from build123d import *

# Parameters (mm, degrees)
SKIZZE1_W                       = 155
SKIZZE1_H                       = 18
AUFSATZ_LINEAR_AUSTRAGEN1_DEPTH = 4
SCHNITT_LINEAR_AUSTRAGEN1_DEPTH = 4
LINEARES_MUSTER1_COUNT          = 22
LINEARES_MUSTER1_PITCH          = 6.379656485
SCHNITT_LINEAR_AUSTRAGEN2_REACH = 6
SKIZZE3_W                       = 115
SKIZZE3_H                       = 4.1
SCHNITT_LINEAR_AUSTRAGEN3_REACH = 6
SKIZZE4_W                       = 3.6
SKIZZE4_H                       = 5


with BuildPart() as part:
    # Skizze1 → Aufsatz-Linear austragen1 (new body)
    with BuildSketch(Plane.XY):
        with Locations((77.5, 9)):
            Rectangle(SKIZZE1_W, SKIZZE1_H)
    extrude(amount=AUFSATZ_LINEAR_AUSTRAGEN1_DEPTH)

    # Skizze2 → Schnitt-Linear austragen1 (cut)
    with BuildSketch(Plane.XY.offset(4)):
        Polygon((0, 13), (1, 13), (2.819851171, 18), (0, 18), align=None)
        Polygon((3.819851171, 18), (5.639702343, 13), (6.639702343, 13), (6.639702343, 18), align=None)
    schnitt_linear_austragen1 = extrude(amount=-SCHNITT_LINEAR_AUSTRAGEN1_DEPTH, mode=Mode.SUBTRACT)

    # Lineares Muster1: Schnitt-Linear austragen1 ×22
    with Locations(*[(i * LINEARES_MUSTER1_PITCH, 0, 0) for i in range(1, LINEARES_MUSTER1_COUNT)]):
        add(schnitt_linear_austragen1, mode=Mode.SUBTRACT)

    # Skizze3 → Schnitt-Linear austragen2 (cut, up to next)
    with BuildSketch(Plane.XY.offset(4), mode=Mode.PRIVATE) as schnitt_linear_austragen2_sk1:
        with Locations((64.227564671, 6.05)):
            Rectangle(SKIZZE3_W, SKIZZE3_H)
    schnitt_linear_austragen2_tool1 = extrude(schnitt_linear_austragen2_sk1.sketch, amount=-SCHNITT_LINEAR_AUSTRAGEN2_REACH, mode=Mode.PRIVATE) & part.part
    add(schnitt_linear_austragen2_tool1.solids().sort_by_distance((64.227565, 6.05, 4))[0], mode=Mode.SUBTRACT)

    # Skizze4 → Schnitt-Linear austragen3 (cut, up to next)
    with BuildSketch(Plane.XY.offset(4), mode=Mode.PRIVATE) as schnitt_linear_austragen3_sk1:
        with Locations((149.2, 15.5)):
            Rectangle(SKIZZE4_W, SKIZZE4_H)
    schnitt_linear_austragen3_tool1 = extrude(schnitt_linear_austragen3_sk1.sketch, amount=-SCHNITT_LINEAR_AUSTRAGEN3_REACH, mode=Mode.PRIVATE) & part.part
    add(schnitt_linear_austragen3_tool1.solids().sort_by_distance((149.2, 15.5, 4))[0], mode=Mode.SUBTRACT)
    # Skizze4 → Schnitt-Linear austragen3 (cut, up to next)
    with BuildSketch(Plane.XY.offset(4), mode=Mode.PRIVATE) as schnitt_linear_austragen3_sk2:
        with Locations((149.2, 2.5)):
            Rectangle(SKIZZE4_W, SKIZZE4_H)
    schnitt_linear_austragen3_tool2 = extrude(schnitt_linear_austragen3_sk2.sketch, amount=-SCHNITT_LINEAR_AUSTRAGEN3_REACH, mode=Mode.PRIVATE) & part.part
    add(schnitt_linear_austragen3_tool2.solids().sort_by_distance((149.2, 2.5, 4))[0], mode=Mode.SUBTRACT)


solid = part.part
Here's how the part is built. I have some questions about the finished solid (model axes, mm). A direction names the side the tool comes from. Coordinates: 2 decimals unless noted, no trailing zeros. Answer in a Markdown table with one row per item.
(1) Please list where these lines run through material, in increasing order: probe 1 along Y at (x, z) = (38.5, 0.3); probe 2 along X at (y, z) = (3, 2.7); probe 3 along X at (y, z) = (7.75, 0.65).
Answer key:
| item | result |
|---|---|
| probe 1 | 0 to 4, 8.1 to 13 |
| probe 2 | 0 to 147.4, 151 to 155 |
| probe 3 | 0 to 6.73, 121.73 to 155 |
(2) On a 3-axis mill with a long thin cutter (end or side, diameter ignored), from which of +Z, -Z, +X, -X, +Y, -Y can I reach the whole of each face in a straight line? I mean faces 1 (the face through (149, 5, 2)), 2 (the face through (73, 0, 2)), 3 (the face through (121.728, 6, 2)), 4 (the face through (147.4, 15, 2)). Say none if no direction works.
Answer key:
| item | result |
|---|---|
| face 1 | +Z, -Z, -Y |
| face 2 | +Z, -Z, +X, -X, -Y |
| face 3 | +Z, -Z |
| face 4 | +Z, -Z, +Y |
(3) Will these pins go through, and if not, where does the flat tip stop? pin 1 Ø1.5 at (x, z) = (133.5, 3.5) entering from -Y; pin 2 Ø0.5 at (x, z) = (134.5, 1) entering from +Y.
Answer key:
| item | result |
|---|---|
| pin 1 | y = 0 |
| pin 2 | y = 13 |
(4) Thinking about a two-plate mould opening in X: for faces 5 (the face through (153, 0, 2)), 6 (the face through (52.934, 15.465, 2.028)), 7 (the face through (0, 6, 2)), which applies, +X half, -X half, draft (parallel to the pull), parting line (faces both ways), or undercut?
Answer key:
| item | result |
|---|---|
| face 5 | draft |
| face 6 | undercut |
| face 7 | -X half |
